Can you work these out from the drawing? Everything is in mm from the part's minimum corner. Coordinates: 2 decimals unless noted, no trailing zeros. Write each loop counter-clockwise with the first axis right and the second up, starting at its lowest first coordinate (ties: lowest second). Pieces come first, ordered by that corner, then holes. Notation, with made-up numbers: (4.25, 79) -> (8.25, 79) arc R29 cw to (8.25, 113) -> close; hole circle Ø1 at (33.5, 41). An arc over 180 degrees is marked (long way). Use a Markdown table: item, result. Add a question column.
Item 1: If I drill on line 1 along X through (y, z) = (10.5, 112.5); line 2 along Z through (x, y) = (42.5, 12.25), over which ranges is the centre line in solid material (lowest first)? Write a range as from..to.
Item 2: Imagine slicing it at A-A, the plane x = 60. Write out the boundary of the cut face in (y, z), and give its area (3 significant figures).
Item 3: Imagine slicing it at B-B, the plane y = 14.25. Write out the boundary of the cut face in (x, z), and give its area (3 significant figures).
Item 4: Will this pin go through, and if not, where does the flat tip stop? pin 1 Ø6.5 at (x, z) = (7.5, 7.5) entering from +Y.
Item 5: Imagine slicing it at C-C, the plane z = 7.5. Write out the boundary of the cut face in (x, y).
Item 6: If we mould it in two halves opening along X, with no side actions, what happens to the marked faces 1, 2 and 3? For each: pulls with the +X half, pulls with the -X half, needs draft (parallel to the pull), parting line crosses it, or undercut.
Item 7: Imagine slicing it at D-D, the plane z = 22.5. Write out the boundary of the cut face in (x, y), and give its area (3 significant figures).
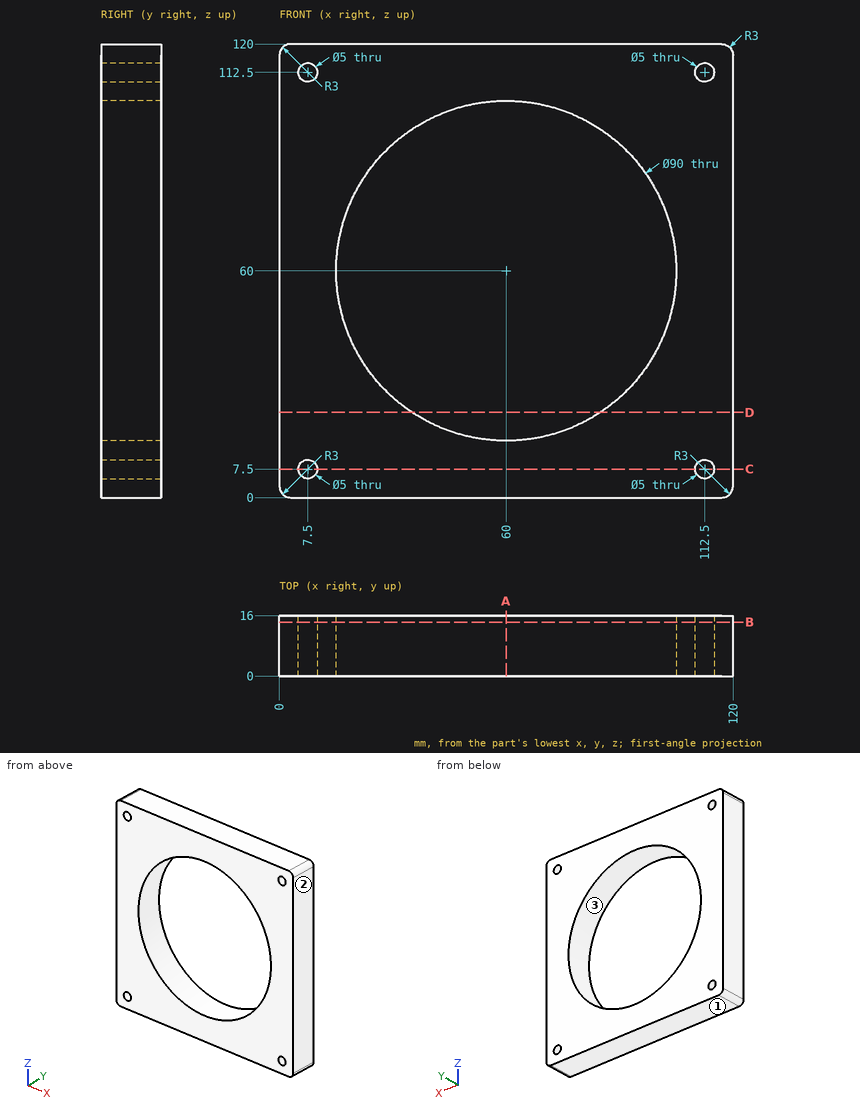
Ans:
| question | item | result |
|---|---|---|
| 1 | line 1 | x = 0..5, 10..110, 115..120 |
| 1 | line 2 | z = 0..18.54, 101.46..120 |
| 2 | outline | (0, 0) -> (16, 0) -> (16, 15) -> (0, 15) -> close; (0, 105) -> (16, 105) -> (16, 120) -> (0, 120) -> close |
| 2 | area | 480 mm^2 |
| 3 | outline | (0, 3) arc R3 ccw to (3, 0) -> (117, 0) arc R3 ccw to (120, 3) -> (120, 117) arc R3 ccw to (117, 120) -> (3, 120) arc R3 ccw to (0, 117) -> close; hole circle Ø5 at (7.5, 7.5); hole circle Ø5 at (7.5, 112.5); hole circle Ø90 at (60, 60); hole circle Ø5 at (112.5, 7.5); hole circle Ø5 at (112.5, 112.5) |
| 3 | area | 7,950 mm^2 |
| 4 | pin 1 | stops at y = 16 |
| 5 | outline | (0, 0) -> (5, 0) -> (5, 16) -> (0, 16) -> close; (10, 0) -> (110, 0) -> (110, 16) -> (10, 16) -> close; (115, 0) -> (120, 0) -> (120, 16) -> (115, 16) -> close |
| 6 | face 1 | needs draft |
| 6 | face 2 | pulls with the +X half |
| 6 | face 3 | undercut |
| 7 | outline | (0, 0) -> (35.13, 0) -> (35.13, 16) -> (0, 16) -> close; (84.87, 0) -> (120, 0) -> (120, 16) -> (84.87, 16) -> close |
| 7 | area | 1,120 mm^2 |
